```python
from build123d import *

# Parameters (mm, degrees)
MODEL_W             = 16.001999145
MODEL_H             = 13.385799247
BOSS_EXTRUDE1_DEPTH = 3.048


with BuildPart() as part:
    # Model → Boss-Extrude1 (new body)
    with BuildSketch(Plane.XY):
        with BuildLine():
            Line((3.047999926, 15.63479994), (0, 15.63479994))
            Line((0, 15.63479994), (0, 5.17))
            Line((0, 5.17), (9.382999755, 5.17))
            Line((9.382999755, 5.17), (9.382999755, 1.5))
            ThreePointArc((9.382999755, 1.5), (9.822339583, 0.439339828), (10.882999755, 0))
            Line((10.882999755, 0), (51.346999833, 0))
            ThreePointArc((51.346999833, 0), (52.407660005, 0.439339828), (52.846999833, 1.5))
            Line((52.846999833, 1.5), (52.846999833, 5.17))
            Line((52.846999833, 5.17), (62.229999341, 5.17))
            Line((62.229999341, 5.17), (62.229999341, 15.63479994))
            Line((62.229999341, 15.63479994), (59.182000346, 15.63479994))
            Line((59.182000346, 15.63479994), (59.182000346, 26.150399451))
            Line((59.182000346, 26.150399451), (57.886601426, 26.150399451))
            Line((57.886601426, 26.150399451), (57.886601426, 10.402400144))
            Line((57.886601426, 10.402400144), (42.392601259, 10.402400144))
            Line((42.392601259, 10.402400144), (42.392601259, 26.150399451))
            Line((42.392601259, 26.150399451), (39.954201318, 26.150399451))
            Line((39.954201318, 26.150399451), (39.954201318, 10.402400144))
            Line((39.954201318, 10.402400144), (24.460199289, 10.402400144))
            Line((24.460199289, 10.402400144), (24.460199289, 26.150399451))
            Line((24.460199289, 26.150399451), (3.047999926, 26.150399451))
            Line((3.047999926, 26.150399451), (3.047999926, 15.63479994))
        make_face()
        with Locations((13.588999515, 16.587299626)):
            Rectangle(MODEL_W, MODEL_H, mode=Mode.SUBTRACT)
    extrude(amount=BOSS_EXTRUDE1_DEPTH)


solid = part.part
```
Build history of the part. All positions in model axes, mm. A direction names the side the tool comes from. Round coordinates to 2 decimals unless told otherwise and drop trailing zeros. Write each loop counter-clockwise with the first axis right and the second up, starting at its lowest first coordinate (ties: lowest second). Pieces come first, ordered by that corner, then holes. Notation, with made-up numbers: (15, 28) -> (52, 28) arc R21 ccw to (52, 58) -> close; hole circle Ø6 at (54.25, -28.75). An arc over 180 degrees is marked (long way). Put each result on its own line as item: value.
Item 1: Tool access for faces 1 (the face through (13, 23.28, 2)), 2 (the face through (9.383, 3, 2)), 3 (the face through (57, 5.17, 2)), 4 (the face through (59.182, 21, 2)): list every direction of +Z, -Z, +X, -X, +Y, -Y with a clear straight run to the whole face (end or side of a thin tool).
Here are the results:
face 1: +Z, -Z
face 2: +Z, -Z, -X, -Y
face 3: +Z, -Z, +X, -Y
face 4: +Z, -Z, +X, +Y
Item 2: Slice it at D-D, the plane y = 12.25. Give the cut face in (x, z), plus the area to 3 significant figures.
Here are the results:
outline: (0, 0) -> (5.59, 0) -> (5.59, 3.05) -> (0, 3.05) -> close; (21.59, 0) -> (24.46, 0) -> (24.46, 3.05) -> (21.59, 3.05) -> close; (39.95, 0) -> (42.39, 0) -> (42.39, 3.05) -> (39.95, 3.05) -> close; (57.89, 0) -> (62.23, 0) -> (62.23, 3.05) -> (57.89, 3.05) -> close
area: 46.5 mm^2
Item 3: Flat gauge pins, fed straight in: P1, Ø1, axis at x = 39.5, y = 16, coming from the -Z side; P2, Ø0.9, axis at x = 36, z = 2, coming from the +Y side; P3, Ø0.9, axis at x = 56, z = 1.5, coming from the -Y side; P4, Ø0.9, axis at y = 21.5, z = 1.5, coming from the +X side. Where does each tip first touch, or does it go through?
Here are the results:
P1: stops at z = 0
P2: stops at y = 10.4
P3: stops at y = 5.17
P4: stops at x = 59.18
Item 4: Slice it at A-A, the plane y = 18.5. Give the cut face in (x, z), plus the area to 3 significant figures.
Here are the results:
outline: (3.05, 0) -> (5.59, 0) -> (5.59, 3.05) -> (3.05, 3.05) -> close; (21.59, 0) -> (24.46, 0) -> (24.46, 3.05) -> (21.59, 3.05) -> close; (39.95, 0) -> (42.39, 0) -> (42.39, 3.05) -> (39.95, 3.05) -> close; (57.89, 0) -> (59.18, 0) -> (59.18, 3.05) -> (57.89, 3.05) -> close
area: 27.9 mm^2
Item 5: Wall check: probe 1 along X at (y, z) = (13.25, 1.55); probe 2 along X at (y, z) = (18.5, 2.15); probe 3 along X at (y, z) = (24.5, 1.6). Give the ranges that are in metal, low to high. Write a range as from..to.
Here are the results:
probe 1: x = 0..5.59, 21.59..24.46, 39.95..42.39, 57.89..62.23
probe 2: x = 3.05..5.59, 21.59..24.46, 39.95..42.39, 57.89..59.18
probe 3: x = 3.05..24.46, 39.95..42.39, 57.89..59.18
Item 6: Slice it at C-C, the plane z = 1.4. Give the cut face in (x, y).
Here are the results:
outline: (0, 5.17) -> (9.38, 5.17) -> (9.38, 1.5) arc R1.5 ccw to (10.88, 0) -> (51.35, 0) arc R1.5 ccw to (52.85, 1.5) -> (52.85, 5.17) -> (62.23, 5.17) -> (62.23, 15.63) -> (59.18, 15.63) -> (59.18, 26.15) -> (57.89, 26.15) -> (57.89, 10.4) -> (42.39, 10.4) -> (42.39, 26.15) -> (39.95, 26.15) -> (39.95, 10.4) -> (24.46, 10.4) -> (24.46, 26.15) -> (3.05, 26.15) -> (3.05, 15.63) -> (0, 15.63) -> close; hole (5.59, 9.89) -> (21.59, 9.89) -> (21.59, 23.28) -> (5.59, 23.28) -> close
Item 7: Two-plate mould, pull along Y, no slides. Class faces 5 (the face through (62.23, 10, 2)), 6 (the face through (31, 0, 2)), 7 (the face through (61, 15.635, 2)), 8 (the face through (5.588, 16, 2)): pulls with the +Y half, pulls with the -Y half, needs draft (parallel to the pull), parting line crosses it, or undercut.
Here are the results:
face 5: needs draft
face 6: pulls with the -Y half
face 7: pulls with the +Y half
face 8: undercut
Item 8: Slice it at B-B, the plane x = 21. Give the cut face in (y, z).
Here are the results:
outline: (0, 0) -> (9.89, 0) -> (9.89, 3.05) -> (0, 3.05) -> close; (23.28, 0) -> (26.15, 0) -> (26.15, 3.05) -> (23.28, 3.05) -> close
